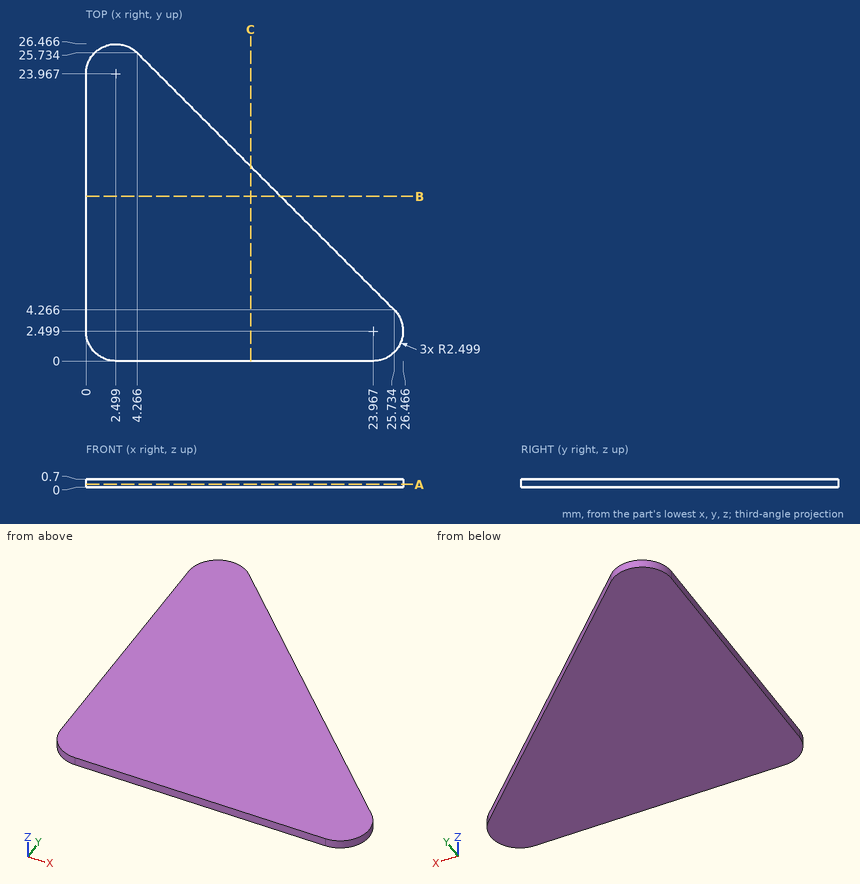
Check sheet for the drawn part. Datum: minimum x, y, z corner. Units: mm. Give positions to 0.01 mm unless a question says otherwise; leave off trailing zeros. Write each loop counter-clockwise with the first axis right and the second up, starting at its lowest first coordinate (ties: lowest second). Pieces come first, ordered by that corner, then holes. Notation, with made-up numbers: (2.25, 46) -> (17.25, 46) arc R25 ccw to (17.25, 62) -> close; hole circle Ø1 at (49.25, 24). An arc over 180 degrees is marked (long way). Use one line per item in the form item = value. Start each with the question number.
1. Section check A-A (z = 0.25). Record the cut outline in (x, y).
2. Section check B-B (y = 13.75). Record the cut outline in (x, z), and give its area (3 significant figures).
3. Thickness scan on line 1 along Y through (x, z) = (8.5, 0.55); line 2 along Y through (x, z) = (24.25, 0.65); line 3 along X through (y, z) = (16.5, 0.6). Record the ranges inside material, lowest first. Write a range as from..to.
4. Go/stop test with a flat-tipped pin: P1, Ø10, axis at x = 13, y = 20.5, coming from the +Z side. Record where the tip stops, or that it passes through.
Conclusion:
q1.outline = (0, 2.5) arc R2.5 ccw to (2.5, 0) -> (23.97, 0) arc R2.5 ccw to (25.73, 4.27) -> (4.27, 25.73) arc R2.5 ccw to (0, 23.97) -> close
q2.outline = (0, 0) -> (16.25, 0) -> (16.25, 0.7) -> (0, 0.7) -> close
q2.area = 11.4 mm²
q3.line_1 = 0..21.5
q3.line_2 = 0.02..5.75
q3.line_3 = 0..13.5
q4.P1 = 0.7
